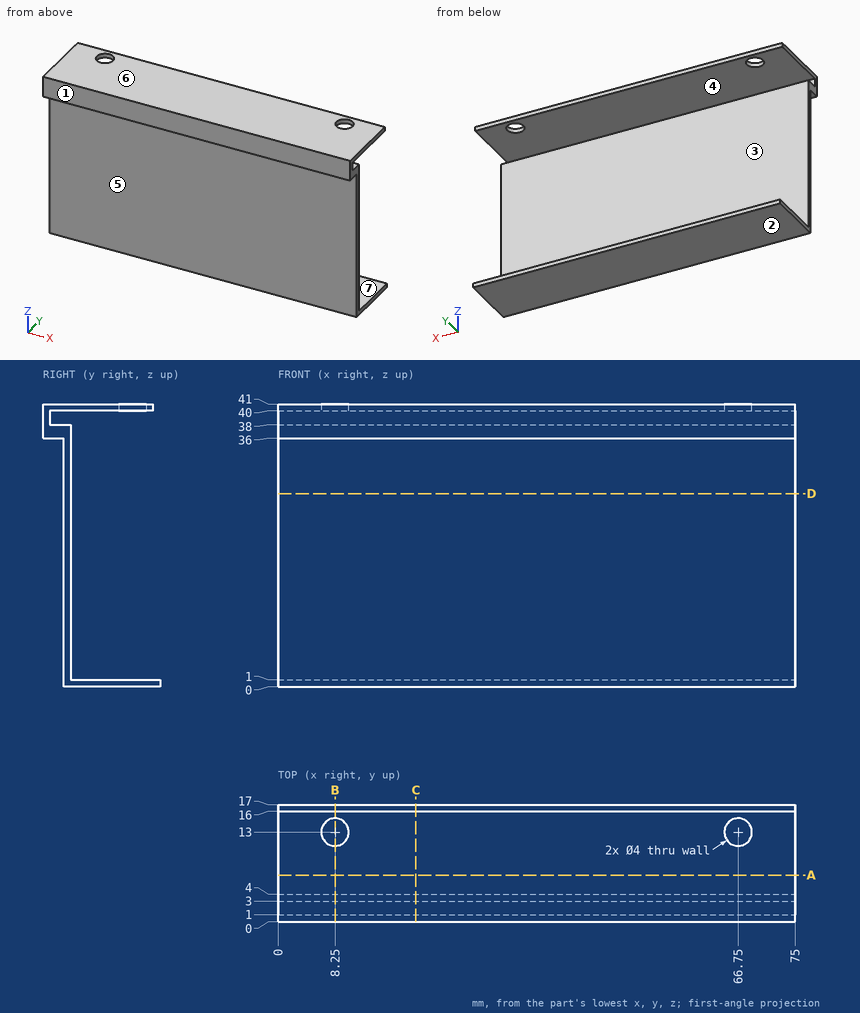
The figure shows three views and two pictorial views of one solid part (mm, origin at its lowest corner). Answer the questions. A direction names the side the tool comes from. Coordinates: 2 decimals unless noted, no trailing zeros. Loops run counter-clockwise (first coordinate to the right, second up) from the corner with the lowest first, then second, coordinate; pieces in that order, holes last. Notation, with made-up numbers: (0.25, 47) -> (40.25, 47) arc R32 cw to (40.25, 73) -> close; hole circle Ø7 at (34, 32.25). An arc over 180 degrees is marked (long way). Write item = value, one per line. Start each with the question number.
1) Given pin 1 Ø0.5 at (x, z) = (49, 40.5) entering from +Y; pin 2 Ø10 at (x, z) = (8, 8.5) entering from -Y; pin 3 Ø0.9 at (x, y) = (45, 1) entering from -Z, each flat-ended and moving along its own axis, determine where each tip first touches the part or whether it passes through.
2) A tool of negligible diameter and unlimited length cuts with its end or side. For the marked faces 5, 6 and 7, from which of +Z, -Z, +X, -X, +Y, -Y can it reach the whole face along a straight path? Write none if from no direction.
3) A cutting plane is placed at B-B (x = 8.25). Give the vertices of the cut face in (y, z), then the cut area to 3 significant figures.
4) The mould has two halves that part along Z. Classify the marked faces 1, 2, 3 and 4: released by +Z, released by -Z, zero draft, split by the parting line, or undercut.
5) A cutting plane is placed at A-A (y = 6.75). Give the vertices of the cut face in (x, z), then the cut area to 3 significant figures.
6) A cutting plane is placed at D-D (z = 28). Give the vertices of the cut face in (x, y).
7) A cutting plane is placed at C-C (x = 20). Give the vertices of the cut face in (y, z).
8) Straight lines are drawn through the part: line 1 (Z direction, x = 60.5, y = 11); line 2 (Z direction, x = 44.5, y = 1.5); line 3 (Y direction, x = 8.25, z = 40.65). For each, find the intervals that lie inside material, in ascending order. Write a range as from..to.
Responses:
q1.pin_1 = 16
q1.pin_2 = 3
q1.pin_3 = 36
q2.face_5 = -Z, +X, -X, -Y
q2.face_6 = +Z, +X, -X, +Y, -Y
q2.face_7 = +X, -X, +Y
q3.outline = (0, 36) -> (3, 36) -> (3, 0) -> (17, 0) -> (17, 1) -> (4, 1) -> (4, 38) -> (1, 38) -> (1, 40) -> (11, 40) -> (11, 41) -> (0, 41) -> close; (15, 40) -> (16, 40) -> (16, 41) -> (15, 41) -> close
q3.area = 71.0 mm²
q4.face_1 = zero draft
q4.face_2 = released by -Z
q4.face_3 = undercut
q4.face_4 = undercut
q5.outline = (0, 0) -> (75, 0) -> (75, 1) -> (0, 1) -> close; (0, 40) -> (75, 40) -> (75, 41) -> (0, 41) -> close
q5.area = 150 mm²
q6.outline = (0, 3) -> (75, 3) -> (75, 4) -> (0, 4) -> close
q7.outline = (0, 36) -> (3, 36) -> (3, 0) -> (17, 0) -> (17, 1) -> (4, 1) -> (4, 38) -> (1, 38) -> (1, 40) -> (16, 40) -> (16, 41) -> (0, 41) -> close
q8.line_1 = 0..1, 40..41
q8.line_2 = 36..38, 40..41
q8.line_3 = 0..11, 15..16
